Build history of the part. All positions in model axes, mm. A direction names the side the tool comes from. Give positions to 0.01 mm unless a question says otherwise; leave off trailing zeros. Loops run counter-clockwise (first coordinate to the right, second up) from the corner with the lowest first, then second, coordinate; pieces in that order, holes last. Notation, with made-up numbers: (79, -1) -> (127, -1) arc R22 cw to (127, 15) -> close; hole circle Ø2 at (12, 86). An arc over 180 degrees is marked (long way). One line per question, with ' | ' between items. Start each with the question number.
(1) Slice it at C-C, the plane x = -39.5. Write the cut outline in (y, z).
(2) Drill centre lines: L1, parallel to X at y = 13, z = 15.5; L2, parallel to X at y = 34.5, z = -44.5; L3, parallel to Z at x = -29, y = -2. Where is each one in solid material? Low to high. Write a range as from..to.
(3) Mould opens along Y. For faces 3 (the face through (-0.65, -7.39, 23.47)), 4 (the face through (0, 0, 0)), 5 (the face through (-26.65, -6.324, -4.032)) say: pulls with the +Y half, pulls with the -Y half, needs draft (parallel to the pull), parting line crosses it, or undercut.
(4) Slice it at A-A, the plane z = 0. Write the cut outline in (x, y), then the cut area to 3 significant figures.
(5) 3-axis set-ups, long thin cutter, end or side, ignore diameter. For faces 1 (the face through (-52, 0, 0)), 2 (the face through (-2, 0, 9)): which of +Z, -Z, +X, -X, +Y, -Y reach the whole face in a straight line?
(6) Flat gauge pins, fed straight in: pin 1 Ø1 at (y, z) = (-33, -8.5) entering from -X; pin 2 Ø5 at (y, z) = (-21, -39) entering from -X; pin 3 Ø5 at (y, z) = (51, -45.5) entering from +X. Where does each tip first touch, or does it go through?
```python
from build123d import *

# Parameters (mm, degrees)
SKETCH_2_R      = 7.5
EXTRUDE_1_DEPTH = 50


with BuildPart() as part:
    # 草图1 → 旋转1 (revolve)
    with BuildSketch(Plane.XY, mode=Mode.PRIVATE) as revolve_1_sk:
        Polygon((0, 0), (0, 20.911534819), (-10.41889066, 80), (-12.388506166, 79.652703645), (-2, 20.736557492), (-2, 0), align=None)
    revolve(revolve_1_sk.sketch.rotate(Axis((-2, 0, 0), (1, 0, 0)), 90), axis=Axis((-2, 0, 0), (1, 0, 0)))

    # 草图2 → 凸台-拉伸1 (add)
    with BuildSketch(Plane.ZY.offset(2)):
        with Locations(Location((0, 0, 0), (0, 0, 180))):
            Circle(SKETCH_2_R)
    extrude(amount=EXTRUDE_1_DEPTH)


solid = part.part
```
Final values:
1) outline: circle Ø15 at (0, 0)
2) L1: -2..0 | L2: -8.27..-6.24 | L3: -7.23..7.23
3) face 3: parting line crosses it | face 4: needs draft | face 5: undercut
4) outline: (-52, -7.5) -> (-2, -7.5) -> (-2, -20.74) -> (-12.39, -79.65) -> (-10.42, -80) -> (0, -20.91) -> (0, 20.91) -> (-10.42, 80) -> (-12.39, 79.65) -> (-2, 20.74) -> (-2, 7.5) -> (-52, 7.5) -> close | area: 1,070 mm2
5) face 1: +Z, -Z, -X, +Y, -Y | face 2: -X
6) pin 1: x = -4.44 | pin 2: x = -6.59 | pin 3: x = -7.92
